```python
from build123d import *

# Parameters (mm, degrees)
F0_R     = 15.875
F0_R_2   = 9.525
F1_DEPTH = 25.4
F2_DEPTH = 25.4
F3_DEPTH = 12.7
F4_R     = 6.35


with BuildPart() as f1:
    # F0 (on Front) → F1 (new body)
    with BuildSketch(Plane.XZ):
        with BuildLine():
            ThreePointArc((5.9015777881, -27.9589342538), (22.1942358541, -17.998514379), (28.575, 0))
            ThreePointArc((28.575, 0), (22.1942358541, 17.998514379), (5.9015777881, 27.9589342538))
            ThreePointArc((5.9015777881, 27.9589342538), (-28.575, 0), (5.9015777881, -27.9589342538))
        make_face()
        Circle(F0_R, mode=Mode.SUBTRACT)
        with BuildLine():
            ThreePointArc((5.9015777881, 27.9589342538), (22.1942358541, 17.998514379), (28.575, 0))
            ThreePointArc((28.575, 0), (22.1942358541, -17.998514379), (5.9015777881, -27.9589342538))
            Line((5.9015777881, -27.9589342538), (48.6725341, -18.9308316998))
            ThreePointArc((48.6725341, -18.9308316998), (31.75, 0), (48.6725341, 18.9308316998))
            Line((48.6725341, 18.9308316998), (5.9015777881, 27.9589342538))
        make_face()
        with BuildLine():
            ThreePointArc((69.85, 0), (63.4959496416, 14.2026533682), (48.6725341, 18.9308316998))
            ThreePointArc((48.6725341, 18.9308316998), (31.75, 0), (48.6725341, -18.9308316998))
            ThreePointArc((48.6725341, -18.9308316998), (63.4959496416, -14.2026533682), (69.85, 0))
        make_face()
        with Locations((50.8, 0)):
            Circle(F0_R_2, mode=Mode.SUBTRACT)
    extrude(amount=-F1_DEPTH)

    # F0 (on Front) → F2 (join)
    with BuildSketch(Plane.XZ):
        with BuildLine():
            ThreePointArc((5.9015777881, -27.9589342538), (22.1942358541, -17.998514379), (28.575, 0))
            ThreePointArc((28.575, 0), (22.1942358541, 17.998514379), (5.9015777881, 27.9589342538))
            ThreePointArc((5.9015777881, 27.9589342538), (-28.575, 0), (5.9015777881, -27.9589342538))
        make_face()
        Circle(F0_R, mode=Mode.SUBTRACT)
    extrude(amount=F2_DEPTH)

    # F0 (on Front) → F3 (cut)
    with BuildSketch(Plane.XZ):
        with BuildLine():
            ThreePointArc((69.85, 0), (63.4959496416, 14.2026533682), (48.6725341, 18.9308316998))
            ThreePointArc((48.6725341, 18.9308316998), (31.75, 0), (48.6725341, -18.9308316998))
            ThreePointArc((48.6725341, -18.9308316998), (63.4959496416, -14.2026533682), (69.85, 0))
        make_face()
        with Locations((50.8, 0)):
            Circle(F0_R_2, mode=Mode.SUBTRACT)
    extrude(amount=-F3_DEPTH, mode=Mode.SUBTRACT)

    # F4
    f4_edges = [f1.edges().sort_by_distance(p)[0] for p in [
        (48.672534, 6.35, -18.930832),
        (48.672534, 6.35, 18.930832),
    ]]
    fillet(f4_edges, radius=F4_R)


solid = f1.part
```
For this review, take the finished solid that the model builds, in its own axes (mm). A direction names the side the tool comes from. Round coordinates to 2 decimals unless told otherwise and drop trailing zeros. Loops run counter-clockwise (first coordinate to the right, second up) from the corner with the lowest first, then second, coordinate; pieces in that order, holes last.
(1) We need section A-A (x = 0). Give the boundary of the cut face in (y, z) (3 decimals).
Returned:
outline: (-25.4, -28.575) - (25.4, -28.575) - (25.4, -15.875) - (-25.4, -15.875) - close; (-25.4, 15.875) - (25.4, 15.875) - (25.4, 28.575) - (-25.4, 28.575) - close
(2) Mouldability with a two-part tool opening along X and no side actions: class faces 1 (the cylindrical face through (59.6, 18.96, -3.65)), 2 (the flat face through (42, 12.7, 5)), 3 (the cylindrical face through (37.143, 6.439, 18.32)) as released by +X, released by -X, zero draft, split by the parting line, or undercut.
Returned:
face 1: undercut
face 2: zero draft
face 3: released by +X
(3) We need section B-B (y = 8.5). Give the boundary of the cut face in (x, z) (3 decimals).
Returned:
outline: (5.902, -27.959) - (32.493, -22.346) arc R6.35 ccw to (36.086, -12.1) arc R19.05 cw to (36.086, 12.1) arc R6.35 ccw to (32.493, 22.346) - (5.902, 27.959) arc R28.575 ccw (long way) to start; hole circle Ø31.75 at (0, 0)
(4) Wall thickness on line 1 along Z through (x, y) = (0, 15) (3 decimals); line 2 along Z through (x, y) = (50.8, 19.75) (3 decimals); line 3 along X through (y, z) = (-7.5, 1.5): over which ranges is each line inside the solid? List them lowest first.
Returned:
line 1: z = -28.575 to -15.875, 15.875 to 28.575
line 2: z = -19.05 to -9.525, 9.525 to 19.05
line 3: x = -28.54 to -15.8, 15.8 to 28.54
(5) Clearance check with flat-ended pins moving along their axes: P1, Ø10, axis at y = -9.5, z = -20, coming from the +X side; P2, Ø1.5, axis at x = 35.5, z = -22, coming from the -Y side; P3, Ø8, axis at y = -10, z = 19.5, coming from the -X side. State where each tip first meets the part, or that it passes through.
Returned:
P1: stops at x = 24.32
P2: stops at y = 12.7
P3: stops at x = -24.01
(6) We need section D-D (z = 4.5). Give the boundary of the cut face in (x, y).
Returned:
outline: (-28.22, -25.4) - (-15.22, -25.4) - (-15.22, 25.4) - (-28.22, 25.4) - close; (15.22, -25.4) - (28.22, -25.4) - (28.22, 0) - (32.29, 0) - (32.29, 12.7) - (42.41, 12.7) - (42.41, 25.4) - (15.22, 25.4) - close; (59.19, 12.7) - (69.31, 12.7) - (69.31, 25.4) - (59.19, 25.4) - close
(7) Tool access review of faces 4 (the flat face through (20, 25.4, 0)), 5 (the cylindrical face through (31.75, 6.26, 0.18)): name each direction out of +Z, -Z, +X, -X, +Y, -Y from which nothing blocks a thin tool from reaching the whole face with its end or side.
Returned:
face 4: +Z, -Z, +X, -X, +Y
face 5: +X, -Y
(8) We need section C-C (y = 21). Give the boundary of the cut face in (x, z) (3 decimals), plus the area to 3 significant figures.
Returned:
outline: (5.902, -27.959) - (48.673, -18.931) arc R19.05 ccw (long way) to (48.673, 18.931) - (5.902, 27.959) arc R28.575 ccw (long way) to start; hole circle Ø31.75 at (0, 0); hole circle Ø19.05 at (50.8, 0)
area: 3,200 mm2
